```python
from build123d import *

# Parameters (mm, degrees)
SKETCH1_W           = 108
SKETCH1_H           = 15
BOSS_EXTRUDE1_DEPTH = 1.5
SKETCH2_W           = 3.202930222
SKETCH2_H           = 8.636913893
BOSS_EXTRUDE2_DEPTH = 2
SKETCH3_R           = 1.5
CUT_EXTRUDE1_DEPTH  = 2


with BuildPart() as part:
    # Sketch1 → Boss-Extrude1 (new body)
    with BuildSketch(Plane(origin=(0, 0, 0), x_dir=(1, 0, 0), z_dir=(0, 1, 0))):
        with Locations((54, -7.5)):
            Rectangle(SKETCH1_W, SKETCH1_H)
    extrude(amount=BOSS_EXTRUDE1_DEPTH)

    # Sketch2 → Boss-Extrude2 (add)
    with BuildSketch(Plane(origin=(0, 1.5, 0), x_dir=(1, 0, 0), z_dir=(0, 1, 0))):
        with Locations((106.398534889, -7.568326669)):
            Rectangle(SKETCH2_W, SKETCH2_H)
    extrude(amount=BOSS_EXTRUDE2_DEPTH)

    # Sketch3 → Cut-Extrude1 (cut)
    with BuildSketch(Plane(origin=(0, 0, 0), x_dir=(-1, 0, 0), z_dir=(0, -1, 0))):
        with Locations(Location((-3, -7.180959686, 0), (0, 0, 90))):
            Circle(SKETCH3_R)
        with Locations(Location((-60.5, -7.180959686, 0), (0, 0, 90))):
            Circle(SKETCH3_R)
        with Locations(Location((-96.5, -7.180959686, 0), (0, 0, 90))):
            Circle(SKETCH3_R)
    extrude(amount=-CUT_EXTRUDE1_DEPTH, mode=Mode.SUBTRACT)


solid = part.part
```
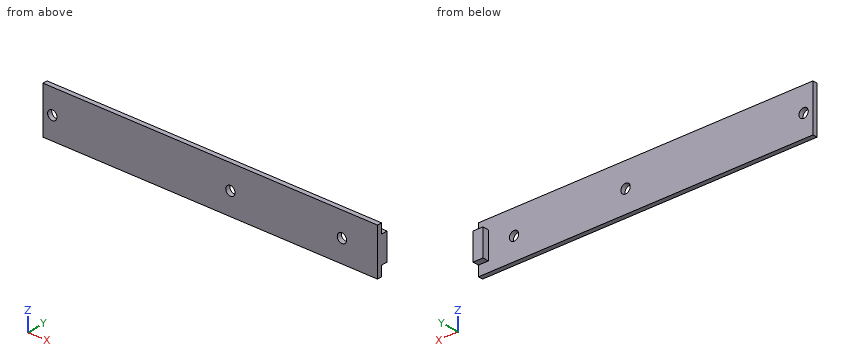
The listing builds one solid part. Answer for the finished solid, in the listing's coordinates (mm). Coordinates: 2 decimals unless noted, no trailing zeros. Loops run counter-clockwise (first coordinate to the right, second up) from the corner with the lowest first, then second, coordinate; pieces in that order, holes last. Notation, with made-up numbers: M -28.5,-39 L -20.5,-39 A21 ccw -20.5,-20 Z; hole C 15.5,70.25 d1. An arc over 180 degrees is marked long. Answer as CSV lines item,"result". Start each with the question number.
(1) Given pin 1 (5 mm diameter, centred on x = 96.5, z = 7.18, fed in from +Y); pin 2 (0.6 mm diameter, centred on x = 105.5, y = 2.5, fed in from +Z); pin 3 (2.5 mm diameter, centred on x = 60.5, z = 7.18, fed in from -Y); pin 4 (1 mm diameter, centred on y = 3, z = 5.5, fed in from -X), each flat-ended and moving along its own axis, determine where each tip first touches the part or whether it passes through.
(2) The part is cut by section C-C (y = 2.4). Give the vertices of the cut face in (x, z), and give its area (3 significant figures).
(3) Find the intervals of material crossed by L1, parallel to X at y = 0.7, z = 7.5; L2, parallel to X at y = 0.3, z = 8.5; L3, parallel to Y at x = 104, z = 14, in increasing order. Write a range as [from, to].
(4) The part is cut by section D-D (x = 37.5). Give the vertices of the cut face in (y, z).
(5) The part is cut by section A-A (x = 60.5). Give the vertices of the cut face in (y, z).
(6) The part is cut by section B-B (z = 9.75). Give the vertices of the cut face in (x, y).
Determined:
1,pin 1,"y = 1.5"
1,pin 2,"z = 11.89"
1,pin 3,"through"
1,pin 4,"x = 104.8"
2,outline,"M 104.8,3.25 L 108,3.25 L 108,11.89 L 104.8,11.89 Z"
2,area,"27.7 mm2"
3,L1,"[0, 1.53], [4.47, 59.03], [61.97, 95.03], [97.97, 108]"
3,L2,"[0, 2.29], [3.71, 59.79], [61.21, 95.79], [97.21, 108]"
3,L3,"[0, 1.5]"
4,outline,"M 0,0 L 1.5,0 L 1.5,15 L 0,15 Z"
5,outline,"M 0,0 L 1.5,0 L 1.5,5.68 L 0,5.68 Z; M 0,8.68 L 1.5,8.68 L 1.5,15 L 0,15 Z"
6,outline,"M 0,0 L 108,0 L 108,3.5 L 104.8,3.5 L 104.8,1.5 L 0,1.5 Z"
